Drawing for the job (mm, zero at the part's lowest x, y, z). A direction names the side the tool comes from. Give positions to 0.01 mm unless a question says otherwise; leave off trailing zeros. Order: outer loops, then holes, each group sorted by start corner. A loop starts at its lowest first (then second) coordinate and runs counter-clockwise, first axis right, second up. Notation, with made-up numbers: (73, 34) - (105, 34) arc R27 cw to (105, 65) - close; hole circle Ø10 at (-18, 62). An arc over 180 degrees is marked (long way). One line per item, written item: value.
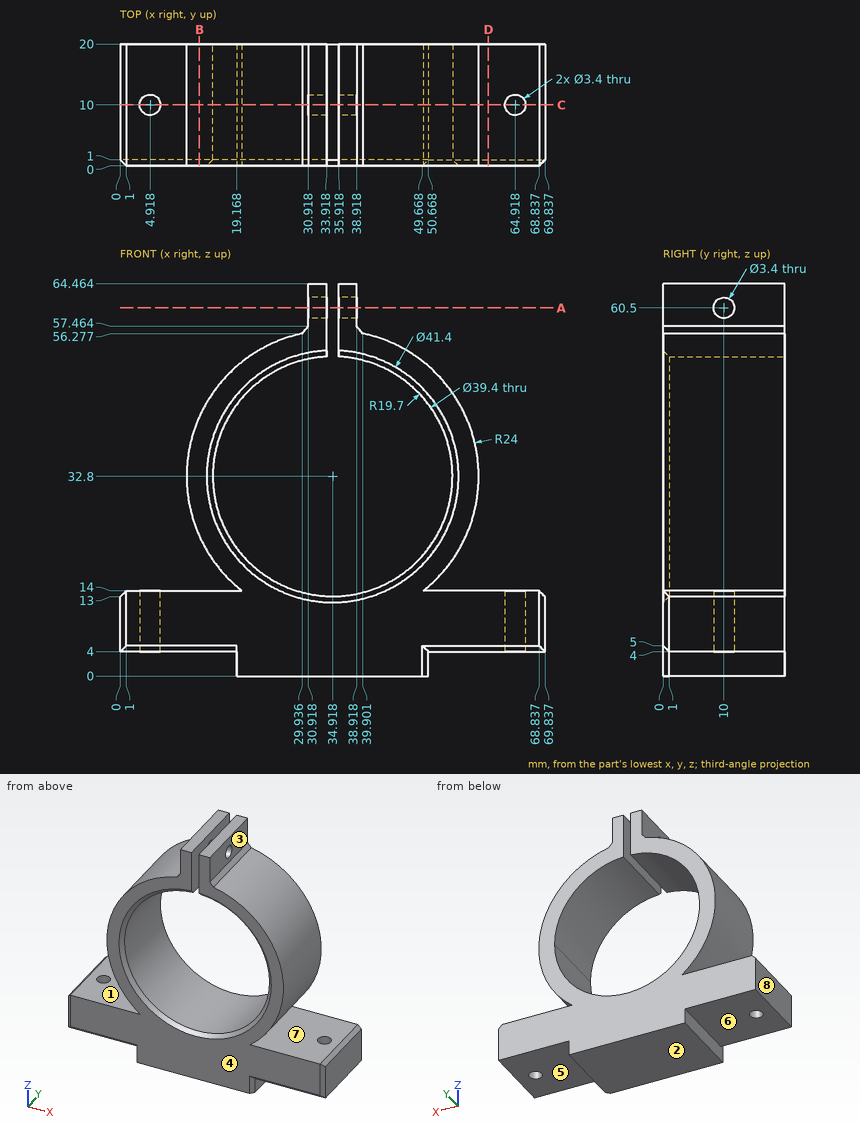
(1) 3-axis set-ups, long thin cutter, end or side, ignore diameter. For the marked faces 4, 5, 6, 7 and 8: which of +Z, -Z, +X, -X, +Y, -Y reach the whole face in a straight line?
Completed:
face 4: +Z, -Z, +X, -X, -Y
face 5: -Z, +X, +Y, -Y
face 6: -Z, -X, +Y, -Y
face 7: +X, +Y, -Y
face 8: +Z, -Z, -X, +Y, -Y
(2) Slice it at B-B, the plane x = 13. Give the cut face in (y, z).
Completed:
outline: (0, 5) - (1, 4) - (20, 4) - (20, 14) - (0, 14) - close; (0, 23.02) - (20, 23.02) - (20, 42.58) - (0, 42.58) - close
(3) Slice it at C-C, the plane y = 10. Count the separate pieces of the cut face and the enclosed holes in it, and give its area (3 significant figures).
Completed:
separate pieces: 5
enclosed holes: 0
area: 1,260 mm²
(4) Drill centre lines: line 1 (X direction, y = 10, z = 12); line 2 (X direction, y = 1, z = 61.5); line 3 (Z direction, x = 36.9, y = 10) (1 decimal). Where is each one in solid material? Low to high.
Completed:
line 1: 0 to 3.22, 6.62 to 63.22, 66.62 to 69.84
line 2: 30.92 to 33.92, 35.92 to 38.92
line 3: 0 to 13.2, 52.4 to 58.8, 62.2 to 64.5
(5) Pin check, flat tips, straight feed: P1, Ø1.5, axis at y = 15, z = 37, coming from the +X side; P2, Ø4, axis at x = 4.92, y = 10, coming from the -Z side; P3, Ø3.5, axis at y = 7, z = 61.5, coming from the +X side; P4, Ø2, axis at y = 10, z = 60.5, coming from the -X side. Stop position of each tip, or through.
Completed:
P1: x = 58.67
P2: z = 4
P3: x = 38.92
P4: through
(6) Pull direction Z, two halves, no side cores. Call the marked faces 1, 2 and 3: +Z half, -Z half, draft (parallel to the pull), parting line (faces both ways), or undercut.
Completed:
face 1: undercut
face 2: -Z half
face 3: draft
(7) Slice it at D-D, the plane x = 60.5. Give the cut face in (y, z).
Completed:
outline: (0, 5) - (1, 4) - (20, 4) - (20, 14) - (0, 14) - close
(8) Slice it at A-A, the plane z = 60.5. Give the cut face in (x, y).
Completed:
outline: (30.92, 0) - (33.92, 0) - (33.92, 8.3) - (30.92, 8.3) - close; (30.92, 11.7) - (33.92, 11.7) - (33.92, 20) - (30.92, 20) - close; (35.92, 0) - (38.92, 0) - (38.92, 8.3) - (35.92, 8.3) - close; (35.92, 11.7) - (38.92, 11.7) - (38.92, 20) - (35.92, 20) - close
